from build123d import *

# Parameters (mm, degrees)
F2_R      = 1.143
F3_DEPTH  = 1.275694
F3_FACE_R = 1.143
F4_DEPTH  = 0.762


with BuildPart() as f1:
    # F0 (on Front) → F1 (revolve)
    with BuildSketch(Plane.XZ):
        with BuildLine():
            ThreePointArc((0, 1.27), (-2.628273, 0.988091), (-5.08, 0))
            Line((-5.08, 0), (-2.38125, 0))
            Line((-2.38125, 0), (-2.38125, -9.525))
            Line((-2.38125, -9.525), (0, -9.525))
            Line((0, -9.525), (0, 1.27))
        make_face()
    revolve(axis=Axis((0, 0, -4.1275), (0, 0, 1)))

    # F2 (on Top) → F3 (cut, through all)
    with BuildSketch(Plane.XY):
        Circle(F2_R)
    extrude(amount=F3_DEPTH, mode=Mode.SUBTRACT)

    # F3_face (on face) → F4 (join)
    with BuildSketch(Plane.XY):
        Circle(F3_FACE_R)
    extrude(amount=F4_DEPTH)


solid = f1.part
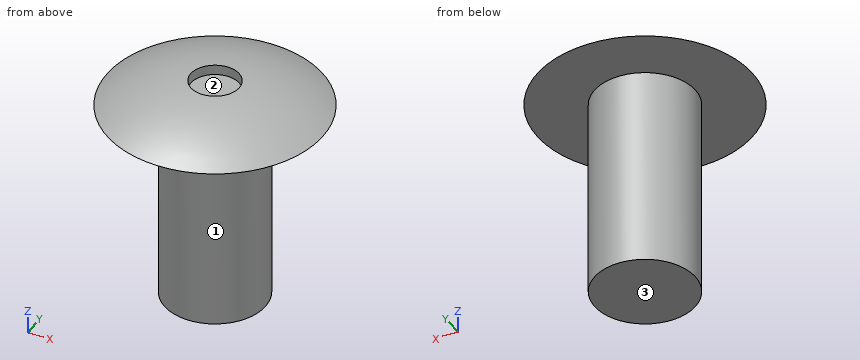
Work out the finished part from the listing and answer in its coordinate system (mm). Face numbers are marked on the shaded views. Round coordinates to 2 decimals unless told otherwise and drop trailing zeros. Write each loop counter-clockwise with the first axis right and the second up, starting at its lowest first coordinate (ties: lowest second). Pieces come first, ordered by that corner, then holes. Notation, with made-up numbers: M 30.25,16 L 73.25,16 A22 cw 73.25,44 Z; hole C -12,48.5 d2. An arc over 180 degrees is marked long. Use a Markdown table: item, result.
1) Determine the mould class of the marked faces 1, 2 and 3 for opening direction X: pulls with the +X half, pulls with the -X half, needs draft (parallel to the pull), parting line crosses it, or undercut.
Taken from the geometry:
| item | result |
|---|---|
| face 1 | parting line crosses it |
| face 2 | undercut |
| face 3 | needs draft |
2) Consider line 1 (Z direction, x = -4.5, y = 1.25); line 2 (Z direction, x = -4, y = 1); line 3 (Y direction, x = -0.5, z = -7.25). Determine where each line is inside the solid, lowest interval first. Write a range as [from, to].
Taken from the geometry:
| item | result |
|---|---|
| line 1 | z = [0, 0.22] |
| line 2 | z = [0, 0.48] |
| line 3 | y = [-2.33, 2.33] |
3) The part is cut by section A-A on z = -6.75. Give the vertices of the cut face in (x, y), plus the area to 3 significant figures.
Taken from the geometry:
| item | result |
|---|---|
| outline | C 0,0 d4.76 |
| area | 17.8 mm2 |
4) Flat-ended cylindrical pins translate along their axes: pin 1 (2 mm diameter, centred on x = -2, z = -5.5, fed in from +Y); pin 2 (2 mm diameter, centred on x = 0, y = 0, fed in from +Z); pin 3 (4 mm diameter, centred on y = -2.5, z = -8, fed in from +X). Find the tip coordinate at first contact, or state that the pin passes through.
Taken from the geometry:
| item | result |
|---|---|
| pin 1 | stops at y = 2.16 |
| pin 2 | stops at z = 0.76 |
| pin 3 | stops at x = 2.33 |
